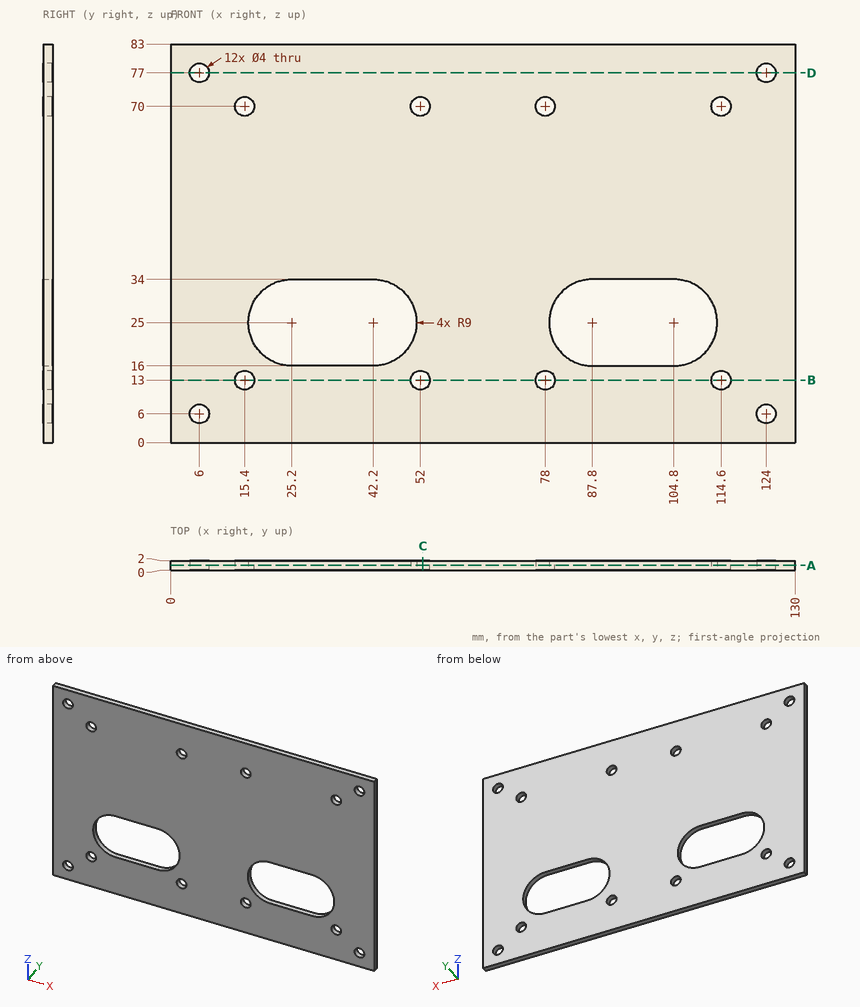
Job drawing, mm, ordinate dimensions from the low corner. One solid piece. Coordinates: 2 decimals unless noted, no trailing zeros. Write each loop counter-clockwise with the first axis right and the second up, starting at its lowest first coordinate (ties: lowest second). Pieces come first, ordered by that corner, then holes.
Item 1: Pin check, flat tip, straight feed: pin 1 (3 mm diameter, centred on x = 78, z = 70, fed in from -Y). Stop position of the tip, or through.
Item 2: Probe line 1 (Z direction, x = 52, y = 0.7); line 2 (X direction, y = 1.45, z = 13); line 3 (X direction, y = 1.5, z = 77). List the from-to ranges inside material, lowest first.
Item 3: Slice it at C-C (x = 52.5). Write the cut outline in (y, z).
Item 4: Slice it at D-D (z = 77). Write the cut outline in (x, y).
Item 5: Slice it at B-B (z = 13). Write the cut outline in (x, y), and give its area (3 significant figures).
Item 6: Slice it at A-A (y = 1). Count the separate pieces of the cut face and the enclosed holes in it, and give its area (3 significant figures).
Results found:
1. pin 1: passes through
2. line 1: z = 0 to 11, 15 to 68, 72 to 83
2. line 2: x = 0 to 13.4, 17.4 to 50, 54 to 76, 80 to 112.6, 116.6 to 130
2. line 3: x = 0 to 4, 8 to 122, 126 to 130
3. outline: (0, 0) - (2, 0) - (2, 11.06) - (0, 11.06) - close; (0, 14.94) - (2, 14.94) - (2, 68.06) - (0, 68.06) - close; (0, 71.94) - (2, 71.94) - (2, 83) - (0, 83) - close
4. outline: (0, 0) - (4, 0) - (4, 2) - (0, 2) - close; (8, 0) - (122, 0) - (122, 2) - (8, 2) - close; (126, 0) - (130, 0) - (130, 2) - (126, 2) - close
5. outline: (0, 0) - (13.4, 0) - (13.4, 2) - (0, 2) - close; (17.4, 0) - (50, 0) - (50, 2) - (17.4, 2) - close; (54, 0) - (76, 0) - (76, 2) - (54, 2) - close; (80, 0) - (112.6, 0) - (112.6, 2) - (80, 2) - close; (116.6, 0) - (130, 0) - (130, 2) - (116.6, 2) - close
5. area: 228 mm2
6. separate pieces: 1
6. enclosed holes: 14
6. area: 9,520 mm2
